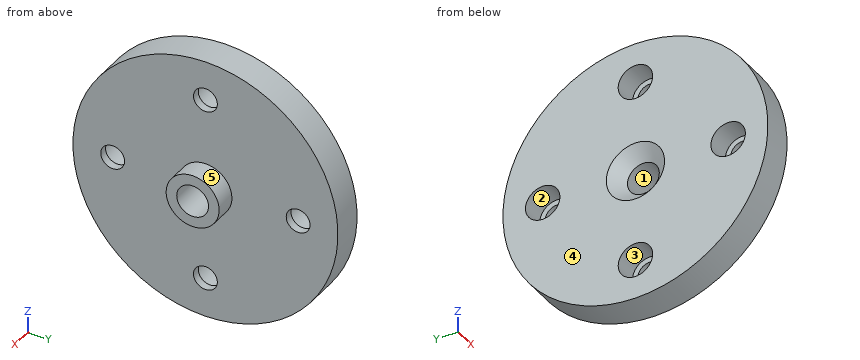
from build123d import *

# Parameters (mm, degrees)
F2_R     = 6.5
F2_R_2   = 4.5
F3_DEPTH = 9
F4_DEPTH = 12
F5_COUNT = 4
F5_ANGLE = 270
F6_SIZE  = 5


with BuildPart() as f1:
    # F0 (on Front) → F1 (revolve)
    with BuildSketch(Plane.XZ):
        Polygon((0, 50), (0, 6), (20, 6), (20, 10), (12, 10), (12, 50), align=None)
    revolve(axis=Axis((48.1764731588, 0, 0), (1, 0, 0)))

    # F2 (on face) → F3 (cut)
    with BuildSketch(Plane(origin=(0, 0, 0), x_dir=(0, -1, 0), z_dir=(-1, 0, 0))):
        with Locations((0, 35)):
            Circle(F2_R)
        with Locations((0, 35)):
            Circle(F2_R_2, mode=Mode.SUBTRACT)
    f3 = extrude(amount=-F3_DEPTH, mode=Mode.SUBTRACT)

    # F2 (on face) → F4 (cut)
    with BuildSketch(Plane(origin=(0, 0, 0), x_dir=(0, -1, 0), z_dir=(-1, 0, 0))):
        with Locations((0, 35)):
            Circle(F2_R_2)
    f4 = extrude(amount=-F4_DEPTH, mode=Mode.SUBTRACT)

    # F5: F3, F4 ×4 about axis
    f5_axis = Axis((48.1764731588, 0, 0), (1, 0, 0))
    for i in range(1, F5_COUNT):
        add(f3.rotate(f5_axis, i * F5_ANGLE / (F5_COUNT - 1)), mode=Mode.SUBTRACT)
        add(f4.rotate(f5_axis, i * F5_ANGLE / (F5_COUNT - 1)), mode=Mode.SUBTRACT)

    # F6
    f6_edges = [f1.edges().sort_by_distance(p)[0] for p in [
        (0, 0, -6),
    ]]
    chamfer(f6_edges, length=F6_SIZE)


solid = f1.part
Work out the finished part from the listing and answer in its coordinate system (mm). Face numbers are marked on the shaded views. A direction names the side the tool comes from. Round coordinates to 2 decimals unless told otherwise and drop trailing zeros. Write each loop counter-clockwise with the first axis right and the second up, starting at its lowest first coordinate (ties: lowest second). Pieces come first, ordered by that corner, then holes. Notation, with made-up numbers: (8.5, 39.5) -> (58.5, 39.5) arc R24 ccw to (58.5, 71.5) -> close; hole circle Ø4 at (22, -37.5). An arc over 180 degrees is marked (long way). Answer as CSV lines item,"result". Start each with the question number.
(1) A tool of negligible diameter and unlimited length cuts with its end or side. For the marked faces 1 and 2, from which of +Z, -Z, +X, -X, +Y, -Y can it reach the whole face along a straight path? Write none if from no direction.
(2) The mould has two halves that part along Z. Classify the marked faces 3, 4 and 5: +Z half, -Z half, draft (parallel to the pull), parting line (faces both ways), or undercut.
(3) The part is cut by section A-A, the plane y = 0. Give the number of separate pieces and of enclosed holes in the cut face, then the cut area to 3 significant figures.
(4) The part is cut by section D-D, the plane y = -32. Give the vertices of the cut face in (x, z).
(5) The part is cut by section B-B, the plane x = 2.5. Give the vertices of the cut face in (y, z), then the cut area to 3 significant figures.
(6) Find the intervals of material crossed by probe 1 along Z at (x, y) = (1, 0); probe 2 along Z at (x, y) = (10.15, 0); probe 3 along Y at (x, z) = (8.75, -5), in increasing order.
(7) Each of these flat-tipped pins is pushed along its axis until it touches: pin 1 (3 mm diameter, centred on y = 13.5, z = 39, fed in from +X); pin 2 (6.5 mm diameter, centred on y = 0, z = 32, fed in from -X); pin 3 (5 mm diameter, centred on x = 9, z = 3.5, fed in from -Y). Where does it stop, or does it pass through?
(8) The part is cut by section C-C, the plane z = 35. Give the vertices of the cut face in (x, y).
Output values:
1,face 1,"+X, -X"
1,face 2,"-X"
2,face 3,"undercut"
2,face 4,"draft"
2,face 5,"parting line"
3,separate pieces,"4"
3,enclosed holes,"0"
3,area,"807 mm²"
4,outline,"(0, -38.42) -> (12, -38.42) -> (12, -3.35) -> (9, -3.35) -> (9, -5.77) -> (0, -5.77) -> close; (0, 5.77) -> (9, 5.77) -> (9, 3.35) -> (12, 3.35) -> (12, 38.42) -> (0, 38.42) -> close"
5,outline,"circle Ø100 at (0, 0); hole circle Ø13 at (-35, 0); hole circle Ø17 at (0, 0); hole circle Ø13 at (0, -35); hole circle Ø13 at (0, 35); hole circle Ø13 at (35, 0)"
5,area,"7,100 mm²"
6,probe 1,"z = -50 to -41.5, -28.5 to -10, 10 to 28.5, 41.5 to 50"
6,probe 2,"z = -50 to -39.5, -30.5 to -6, 6 to 30.5, 39.5 to 50"
6,probe 3,"y = -49.75 to -39.15, -30.85 to -3.32, 3.32 to 30.85, 39.15 to 49.75"
7,pin 1,"stops at x = 12"
7,pin 2,"stops at x = 9"
7,pin 3,"stops at y = -49.99"
8,outline,"(0, -35.71) -> (12, -35.71) -> (12, -4.5) -> (9, -4.5) -> (9, -6.5) -> (0, -6.5) -> close; (0, 6.5) -> (9, 6.5) -> (9, 4.5) -> (12, 4.5) -> (12, 35.71) -> (0, 35.71) -> close"
